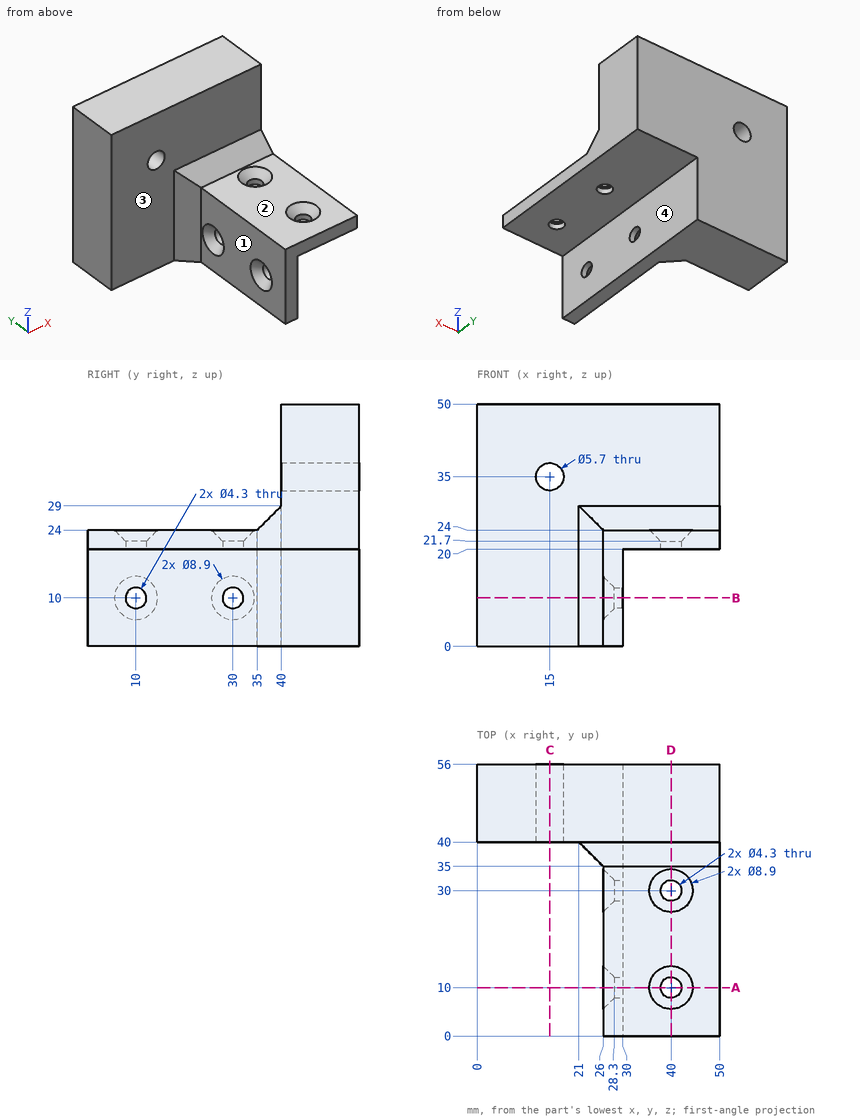
Study the drawing (mm; zero at the part's minimum x, y, z) and answer. A direction names the side the tool comes from. Round coordinates to 2 decimals unless told otherwise and drop trailing zeros. Write each loop counter-clockwise with the first axis right and the second up, starting at its lowest first coordinate (ties: lowest second). Pieces come first, ordered by that corner, then holes. Notation, with made-up numbers: (4, 16) - (41, 16) arc R5 cw to (41, 25) - close; hole circle Ø1 at (82, 78). An arc over 180 degrees is marked (long way). Use a Markdown table: item, result. Add a question column.
1. The part is cut by section B-B (z = 10). Write down the section's boundary in (x, y), and give its area (3 significant figures).
2. The part is cut by section D-D (x = 40). Write down the section's boundary in (y, z).
3. The part is cut by section A-A (y = 10). Write down the section's boundary in (x, z), and give its area (3 significant figures).
4. A tool of negligible diameter and unlimited length cuts with its end or side. For the marked faces 1, 2, 3 and 4, from which of +Z, -Z, +X, -X, +Y, -Y can it reach the whole face along a straight path? Write none if from no direction.
5. Consider line 1 (Y direction, x = 40, z = 21); line 2 (Y direction, x = 28, z = 10); line 3 (Z direction, x = 15, y = 51). Determine where each line is inside the solid, lowest interval first.
6. Flat-ended cylindrical pins translate along their axes: P1, Ø5, axis at y = 30, z = 10, coming from the +X side; P2, Ø4, axis at x = 40, y = 30, coming from the +Z side; P3, Ø6, axis at x = 39.5, y = 23, coming from the -Z side; P4, Ø7, axis at x = 42.5, y = 11, coming from the +Z side. Find the tip coordinate at first contact, or state that the pin passes through.
7. The part is cut by section C-C (x = 15). Write down the section's boundary in (y, z).
Reported:
| question | item | result |
|---|---|---|
| 1 | outline | (0, 40) - (21, 40) - (26, 35) - (26, 34.45) - (28.3, 32.15) - (30, 32.15) - (30, 56) - (0, 56) - close; (26, 0) - (30, 0) - (30, 7.85) - (28.3, 7.85) - (26, 5.55) - close; (26, 14.45) - (28.3, 12.15) - (30, 12.15) - (30, 27.85) - (28.3, 27.85) - (26, 25.55) - close |
| 1 | area | 608 mm^2 |
| 2 | outline | (0, 20) - (7.85, 20) - (7.85, 21.7) - (5.55, 24) - (0, 24) - close; (12.15, 20) - (27.85, 20) - (27.85, 21.7) - (25.55, 24) - (14.45, 24) - (12.15, 21.7) - close; (32.15, 20) - (56, 20) - (56, 50) - (40, 50) - (40, 29) - (35, 24) - (34.45, 24) - (32.15, 21.7) - close |
| 3 | outline | (26, 0) - (30, 0) - (30, 7.85) - (28.3, 7.85) - (26, 5.55) - close; (26, 14.45) - (28.3, 12.15) - (30, 12.15) - (30, 20) - (37.85, 20) - (37.85, 21.7) - (35.55, 24) - (26, 24) - close; (42.15, 20) - (50, 20) - (50, 24) - (44.45, 24) - (42.15, 21.7) - close |
| 3 | area | 131 mm^2 |
| 4 | face 1 | +Z, -Z, -X, -Y |
| 4 | face 2 | +Z, +X, -X, -Y |
| 4 | face 3 | +Z, -X, -Y |
| 4 | face 4 | -Z, +X, +Y, -Y |
| 5 | line 1 | 0 to 7.85, 12.15 to 27.85, 32.15 to 56 |
| 5 | line 2 | 0 to 7.55, 12.45 to 27.55, 32.45 to 56 |
| 5 | line 3 | 0 to 32.15, 37.85 to 50 |
| 6 | P1 | x = 30 |
| 6 | P2 | through |
| 6 | P3 | z = 20 |
| 6 | P4 | z = 24 |
| 7 | outline | (40, 0) - (56, 0) - (56, 32.15) - (40, 32.15) - close; (40, 37.85) - (56, 37.85) - (56, 50) - (40, 50) - close |
